from build123d import *

# Parameters (mm, degrees)
F0_W      = 609.6
F0_H      = 304.8
F1_DEPTH  = 21.971
F2_W      = 596.9
F2_H      = 292.1
F3_DEPTH  = 5.715
F5_W      = 558.8
F5_H      = 203.2
F6_DEPTH  = 27.687
F8_W      = 12.7
F8_H      = 19.431
F9_DEPTH  = 609.601
F10_R     = 38.1
F11_DEPTH = 19.431
F12_R     = 6.35
F13_DEPTH = 8.256
F14_R     = 6.35
F15_DEPTH = 609.601
F16_R     = 6.35
F17_DEPTH = 27.687


with BuildPart() as f1:
    # F0 (on Top) → F1 (new body)
    with BuildSketch(Plane.XY):
        with Locations((304.8, 152.4)):
            Rectangle(F0_W, F0_H)
    extrude(amount=F1_DEPTH)

    # F2 (on face) → F3 (join)
    with BuildSketch(Plane(origin=(0, 0, 0), x_dir=(1, 0, 0), z_dir=(0, 0, -1))):
        with Locations((304.8, -152.4)):
            Rectangle(F2_W, F2_H)
    extrude(amount=F3_DEPTH)

    # F5 (on face) → F6 (cut, through all)
    with BuildSketch(Plane.XY.offset(21.971)):
        with Locations((304.8, 152.4)):
            Rectangle(F5_W, F5_H)
    extrude(amount=-F6_DEPTH, mode=Mode.SUBTRACT)

    # F8 (on face) → F9 (cut, through all)
    with BuildSketch(Plane(origin=(0, 0, 0), x_dir=(0, -1, 0), z_dir=(-1, 0, 0))):
        with Locations((-298.45, 12.2555)):
            Rectangle(F8_W, F8_H)
        with Locations((-6.35, 12.2555)):
            Rectangle(F8_W, F8_H)
    extrude(amount=-F9_DEPTH, mode=Mode.SUBTRACT)

    # F10 (on face) → F11 (cut, through all)
    with BuildSketch(Plane.XY.offset(21.971)):
        with Locations((304.8, 40.64)):
            Circle(F10_R)
        with Locations((304.8, 264.16)):
            Circle(F10_R)
    extrude(amount=-F11_DEPTH, mode=Mode.SUBTRACT)

    # F12 (on face) → F13 (cut, through all)
    with BuildSketch(Plane.XY.offset(2.54)):
        with Locations((304.8, 264.16)):
            Circle(F12_R)
        with Locations((304.8, 40.64)):
            Circle(F12_R)
    extrude(amount=-F13_DEPTH, mode=Mode.SUBTRACT)

    # F14 (on face) → F15 (cut, through all)
    with BuildSketch(Plane.YZ.offset(609.6)):
        with Locations((228.6, 11.811)):
            Circle(F14_R)
        with Locations((76.2, 11.811)):
            Circle(F14_R)
    extrude(amount=-F15_DEPTH, mode=Mode.SUBTRACT)

    # F16 (on face) → F17 (cut, through all)
    with BuildSketch(Plane.XY.offset(21.971)):
        with Locations((368.3, 25.4)):
            Circle(F16_R)
        with Locations((368.3, 279.4)):
            Circle(F16_R)
    extrude(amount=-F17_DEPTH, mode=Mode.SUBTRACT)


solid = f1.part
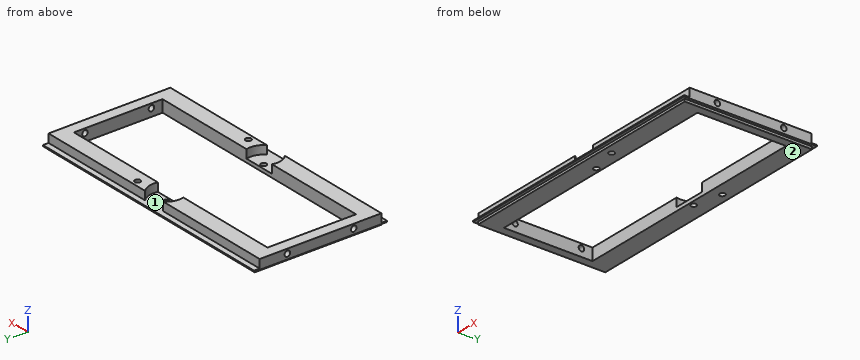
The listing builds one solid part. Answer for the finished solid, in the listing's coordinates (mm). Face numbers are marked on the shaded views. Coordinates: 2 decimals unless noted, no trailing zeros. Write each loop counter-clockwise with the first axis right and the second up, starting at its lowest first coordinate (ties: lowest second). Pieces come first, ordered by that corner, then holes. Notation, with made-up numbers: M 74,13 L 86,13 A22 ccw 86,29 Z; hole C -14.5,-14.75 d7. An arc over 180 degrees is marked long. Put each result on its own line as item: value. Start each with the question number.
1. A cutting plane is placed at D-D on y = 40.64. Write down the section's boundary in (x, z) (3 decimals).
2. A cutting plane is placed at B-B on x = 490. Write down the section's boundary in (y, z) (3 decimals).
3. A cutting plane is placed at A-A on y = 117. Write down the section's boundary in (x, z) (3 decimals), then the cut area to 3 significant figures.
4. A cutting plane is placed at C-C on y = 228.6. Write down the section's boundary in (x, z) (3 decimals), then the cut area to 3 significant figures.
5. Consider line 1 (Y direction, x = 368.3, z = 3); line 2 (X direction, y = 199, z = 9); line 3 (X direction, y = 243.5, z = -2.5). Determine where each line is inside the solid, lowest interval first. Write a range as from..to.
6. Flat-ended cylindrical pins translate along their axes: P1, Ø3, axis at x = 541.5, z = 7, coming from the +Y side; P2, Ø1.7, axis at y = 112, z = -3, coming from the +X side; P3, Ø6.5, axis at y = 188, z = -4, coming from the -X side. Find the tip coordinate at first contact, or state that the pin passes through.
7. For a pull along X with two mould halves and no side action, classify the marked faces 1 and 2 as pulls with the +X half, pulls with the -X half, needs draft (parallel to the pull), parting line crosses it, or undercut.
Resolved:
1. outline: M 0,0 L 6.35,0 L 6.35,-5.715 L 298.45,-5.715 L 298.45,2.54 L 266.7,2.54 L 266.7,21.971 L 0,21.971 Z; M 311.15,-5.715 L 603.25,-5.715 L 603.25,0 L 609.6,0 L 609.6,21.971 L 342.9,21.971 L 342.9,2.54 L 311.15,2.54 Z
2. outline: M 0,0 L 6.35,0 L 6.35,-5.715 L 50.8,-5.715 L 50.8,21.971 L 12.7,21.971 L 12.7,2.54 L 0,2.54 Z; M 254,-5.715 L 298.45,-5.715 L 298.45,0 L 304.8,0 L 304.8,2.54 L 292.1,2.54 L 292.1,21.971 L 254,21.971 Z
3. outline: M 0,0 L 6.35,0 L 6.35,-5.715 L 25.4,-5.715 L 25.4,21.971 L 0,21.971 Z; M 584.2,-5.715 L 603.25,-5.715 L 603.25,0 L 609.6,0 L 609.6,21.971 L 584.2,21.971 Z
3. area: 1,330 mm2
4. outline: M 0,0 L 6.35,0 L 6.35,-5.715 L 25.4,-5.715 L 25.4,5.461 L 0,5.461 Z; M 0,18.161 L 25.4,18.161 L 25.4,21.971 L 0,21.971 Z; M 584.2,-5.715 L 603.25,-5.715 L 603.25,0 L 609.6,0 L 609.6,5.461 L 584.2,5.461 Z; M 584.2,18.161 L 609.6,18.161 L 609.6,21.971 L 584.2,21.971 Z
4. area: 689 mm2
5. line 1: y = 12.7..19.05, 31.75..50.8, 254..273.05, 285.75..292.1
5. line 2: x = 0..25.4, 584.2..609.6
5. line 3: x = 6.35..25.4, 584.2..603.25
6. P1: stops at y = 292.1
6. P2: stops at x = 603.25
6. P3: stops at x = 6.35
7. face 1: undercut
7. face 2: needs draft
